Read the model definition and answer for the solid it produces. Units are mm, in the model's axes. A direction names the side the tool comes from. Coordinates: 2 decimals unless noted, no trailing zeros. Loops run counter-clockwise (first coordinate to the right, second up) from the corner with the lowest first, then second, coordinate; pieces in that order, holes last. Notation, with made-up numbers: (21, -17) - (73, -17) arc R21 ccw to (73, 7) - close; hole circle Ø4 at (71, 80.25). An arc over 180 degrees is marked (long way). One line per question, with ' | ' between items. Start each with the question number.
```python
from build123d import *

# Parameters (mm, degrees)
SKETCH1_W           = 100
SKETCH1_H           = 100
BOSS_EXTRUDE2_DEPTH = 150
CUT_EXTRUDE1_DEPTH  = 80
CUT_EXTRUDE2_DEPTH  = 103
SKETCH3_W           = 60
SKETCH3_H           = 10
CUT_EXTRUDE3_DEPTH  = 178
CUT_EXTRUDE4_DEPTH  = 81
SKETCH5_W           = 60
SKETCH5_H           = 60
SKETCH5_R           = 15
CUT_EXTRUDE5_DEPTH  = 90
SKETCH6_R           = 15
CUT_EXTRUDE6_DEPTH  = 128


with BuildPart() as part:
    # Sketch1 → Boss-Extrude2 (new body)
    with BuildSketch(Plane.XY):
        with Locations((50, 50)):
            Rectangle(SKETCH1_W, SKETCH1_H)
    extrude(amount=-BOSS_EXTRUDE2_DEPTH)

    # Sketch2 → Cut-Extrude1 (cut)
    with BuildSketch(Plane(origin=(0, 100, 0), x_dir=(1, 0, 0), z_dir=(0, 1, 0))):
        with BuildLine():
            Line((100, 35), (0, 35))
            Line((0, 35), (0, 0))
            Line((0, 0), (42.5, 0))
            Line((42.5, 0), (42.5, 15))
            ThreePointArc((42.5, 15), (50, 22.5), (57.5, 15))
            Line((57.5, 15), (57.5, 0))
            Line((57.5, 0), (100, 0))
            Line((100, 0), (100, 35))
        make_face()
        with BuildLine():
            ThreePointArc((57.5, 135), (50, 127.5), (42.5, 135))
            Line((42.5, 135), (42.5, 150))
            Line((42.5, 150), (0, 150))
            Line((0, 150), (0, 115))
            Line((0, 115), (100, 115))
            Line((100, 115), (100, 150))
            Line((100, 150), (57.5, 150))
            Line((57.5, 150), (57.5, 135))
        make_face()
    extrude(amount=-CUT_EXTRUDE1_DEPTH, mode=Mode.SUBTRACT)

    # Sketch2<3> → Cut-Extrude2 (cut)
    with BuildSketch(Plane(origin=(0, 100, 0), x_dir=(1, 0, 0), z_dir=(0, 1, 0))):
        with BuildLine():
            Line((57.5, 0), (57.5, 15))
            ThreePointArc((57.5, 15), (50, 22.5), (42.5, 15))
            Line((42.5, 15), (42.5, 0))
            Line((42.5, 0), (57.5, 0))
        make_face()
        with BuildLine():
            Line((42.5, 150), (42.5, 135))
            ThreePointArc((42.5, 135), (50, 127.5), (57.5, 135))
            Line((57.5, 135), (57.5, 150))
            Line((57.5, 150), (42.5, 150))
        make_face()
    extrude(amount=-CUT_EXTRUDE2_DEPTH, mode=Mode.SUBTRACT)

    # Sketch3 → Cut-Extrude3 (cut)
    with BuildSketch(Plane.XY):
        with Locations((50, 5)):
            Rectangle(SKETCH3_W, SKETCH3_H)
    extrude(amount=-CUT_EXTRUDE3_DEPTH, mode=Mode.SUBTRACT)

    # Sketch4 → Cut-Extrude4 (cut)
    with BuildSketch(Plane.XY.offset(-35)):
        Polygon((100, 100), (20, 100), (100, 40), align=None)
    extrude(amount=-CUT_EXTRUDE4_DEPTH, mode=Mode.SUBTRACT)

    # Sketch5 → Cut-Extrude5 (cut)
    with BuildSketch(Plane(origin=(100, 0, 0), x_dir=(0, 0, -1), z_dir=(1, 0, 0))):
        with Locations((75, 60)):
            Rectangle(SKETCH5_W, SKETCH5_H)
        with Locations((75, 60)):
            Circle(SKETCH5_R, mode=Mode.SUBTRACT)
    extrude(amount=-CUT_EXTRUDE5_DEPTH, mode=Mode.SUBTRACT)

    # Sketch6 → Cut-Extrude6 (cut)
    with BuildSketch(Plane(origin=(100, 0, 0), x_dir=(0, 0, -1), z_dir=(1, 0, 0))):
        with Locations((75, 60)):
            Circle(SKETCH6_R)
    extrude(amount=-CUT_EXTRUDE6_DEPTH, mode=Mode.SUBTRACT)


solid = part.part
```
1) The part is cut by section C-C on y = 60. Write down the section's boundary in (x, z).
2) Given pin 1 Ø5 at (x, z) = (49.5, -77) entering from +Y; pin 2 Ø3 at (x, y) = (38.5, 73.5) entering from -Z; pin 3 Ø12 at (x, z) = (31.5, -122.5) entering from +Y, each flat-ended and moving along its own axis, determine where each tip first touches the part or whether it passes through.
3) The mould has two halves that part along Z. Classify faces 1 (the flat face through (10, 74, -68)), 2 (the flat face through (83, 12, -150)), 3 (the cylindrical face through (5.07, 45.357, -71.748)), 4 (the cylindrical face through (50.16, 15.07, -22.5)): released by +Z, released by -Z, zero draft, split by the parting line, or undercut.
4) The part is cut by section A-A on z = -75. Write down the section's boundary in (x, y).
5) Which of the six approach directions +Z, -Z, +X, -X, +Y, -Y give full straight-line access (tool end or side, diameter ignored) to faces 5 (the flat face through (42.5, 15, -8)), 6 (the flat face through (56, 30, -75)), 7 (the flat face through (40, 52, -35)), 8 (the flat face through (38, 52, -115)), 9 (the flat face through (50, 10, -74))?
6) The part is cut by section D-D on z = -42.5. Write down the section's boundary in (x, y), and give its area (3 significant figures).
7) The part is cut by section B-B on x = 50. Write down the section's boundary in (y, z), and give its area (3 significant figures).
8) Find the intervals of material crossed by line 1 along Z through (x, y) = (22, 44.5); line 2 along X through (y, z) = (6, -13); line 3 along Y through (x, z) = (6, -75), in increasing order. Write a range as from..to.
Answer below:
1) outline: (0, -115) - (73.33, -115) - (73.33, -105) - (10, -105) - (10, -90) - (0, -90) - close; (0, -60) - (10, -60) - (10, -45) - (73.33, -45) - (73.33, -35) - (0, -35) - close
2) pin 1: y = 30 | pin 2: z = -115 | pin 3: y = 20
3) face 1: undercut | face 2: released by -Z | face 3: undercut | face 4: released by +Z
4) outline: (0, 0) - (20, 0) - (20, 10) - (80, 10) - (80, 0) - (100, 0) - (100, 30) - (10, 30) - (10, 45) - (0, 45) - close; (0, 75) - (10, 75) - (10, 90) - (33.33, 90) - (20, 100) - (0, 100) - close
5) face 5: +Z, +Y, -Y | face 6: +X | face 7: +Z, +X, -X, +Y | face 8: -Z, +X, -X, +Y | face 9: +Z, -Z, -Y
6) outline: (0, 0) - (20, 0) - (20, 10) - (80, 10) - (80, 0) - (100, 0) - (100, 40) - (20, 100) - (0, 100) - close | area: 7,000 mm2
7) outline: (10, -127.5) - (20, -127.5) - (20, -115) - (77.5, -115) - (77.5, -105) - (30, -105) - (30, -45) - (77.5, -45) - (77.5, -35) - (20, -35) - (20, -22.5) - (10, -22.5) - close | area: 2,800 mm2
8) line 1: -115..-105, -45..-35 | line 2: 0..20, 80..100 | line 3: 0..45, 75..100
